Read the model definition and answer for the solid it produces. Units are mm, in the model's axes. A direction names the side the tool comes from. Coordinates: 2 decimals unless noted, no trailing zeros. Write each loop counter-clockwise with the first axis right and the second up, starting at its lowest first coordinate (ties: lowest second). Pieces come first, ordered by that corner, then holes. Notation, with made-up numbers: (59, 62) -> (83, 62) arc R6 cw to (83, 71) -> close; hole circle Ø11 at (20.5, 62). An arc over 180 degrees is marked (long way). One line per item, written item: value. Start each with the question number.
1. Consider line 1 along Y through (x, z) = (11, 3.5); line 2 along Y through (x, z) = (3.75, 0.5); line 3 along Z through (x, y) = (-0.75, 14.75). Determine where each line is inside the solid, lowest interval first.
2. Given P1, Ø4, axis at x = -4.5, z = 2, coming from the +Y side; P2, Ø2.5, axis at y = 18, z = 3.5, coming from the +X side; P3, Ø3, axis at x = 7.5, z = 4, coming from the +Y side, each flat-ended and moving along its own axis, determine where each tip first touches the part or whether it passes through.
3. Find section D-D, the plane z = -2. Write down the section's boundary in (x, y).
4. Find section A-A, the plane z = 4. Write down the section's boundary in (x, y).
5. Find section B-B, the plane x = 3. Write down the section's boundary in (y, z), and give its area (3 significant figures).
6. For faces 1 (the flat face through (4.965, 7.465, 2.605)), 2 (the flat face through (-12.5, 10, 0)), determine the directions among +Z, -Z, +X, -X, +Y, -Y from which every point of the face is accessible in a straight line to the end or side of a thin tool.
7. Find section C-C, the plane y = 6. Write down the section's boundary in (x, z), and give its area (4 significant figures).
```python
from build123d import *

# Parameters (mm, degrees)
SKETCH_1_W          = 5
SKETCH_1_H          = 15
EXTRUDE_1_DEPTH     = 5
EXTRUDE_2_DEPTH     = 10
SKETCH_1_4_W        = 5
SKETCH_1_4_H        = 15
EXTRUDE_3_DEPTH     = 15
EXTRUDE_4_DEPTH     = 20
CUT_EXTRUDE_1_DEPTH = 20


with BuildPart() as part:
    # Sketch 1 → Extrude 1 (new body)
    with BuildSketch(Plane(origin=(0, 0, 0), x_dir=(1, 0, 0), z_dir=(0, 1, 0))):
        Polygon((7.5, 5), (12.5, 5), (12.5, 10), (-12.5, 10), (-12.5, -10), (-7.5, -10), (-7.5, 5), (-2.5, 5), align=None)
        with Locations((-5, -2.5)):
            Rectangle(SKETCH_1_W, SKETCH_1_H)
        Polygon((2.5, -10), (7.5, 5), (-2.5, 5), (-2.5, -10), align=None)
        Polygon((12.5, -10), (12.5, 5), (7.5, 5), (2.5, -10), align=None)
    extrude(amount=EXTRUDE_1_DEPTH)

    # Sketch 1_3 → Extrude 2 (add)
    with BuildSketch(Plane(origin=(0, 0, 0), x_dir=(1, 0, 0), z_dir=(0, 1, 0))):
        Polygon((2.5, -10), (7.5, 5), (-2.5, 5), (-2.5, -10), align=None)
    extrude(amount=EXTRUDE_2_DEPTH)

    # Sketch 1_4 → Extrude 3 (add)
    with BuildSketch(Plane(origin=(0, 0, 0), x_dir=(1, 0, 0), z_dir=(0, 1, 0))):
        with Locations((-5, -2.5)):
            Rectangle(SKETCH_1_4_W, SKETCH_1_4_H)
    extrude(amount=EXTRUDE_3_DEPTH)

    # Sketch 1_5 → Extrude 4 (add)
    with BuildSketch(Plane(origin=(0, 0, 0), x_dir=(1, 0, 0), z_dir=(0, 1, 0))):
        Polygon((7.5, 5), (12.5, 5), (12.5, 10), (-12.5, 10), (-12.5, -10), (-7.5, -10), (-7.5, 5), (-2.5, 5), align=None)
    extrude(amount=EXTRUDE_4_DEPTH)

    # Sketch 2 → Cut-Extrude 1 (cut)
    with BuildSketch(Plane.XY.offset(-5)):
        Polygon((12.5, 20), (2.5, 20), (12.5, 10), align=None)
    extrude(amount=-CUT_EXTRUDE_1_DEPTH, mode=Mode.SUBTRACT)


solid = part.part
```
Answer block:
1. line 1: y = 0 to 5
1. line 2: y = 0 to 10
1. line 3: z = -10 to -5
2. P1: stops at y = 15
2. P2: stops at x = -7.5
2. P3: stops at y = 5
3. outline: (-12.5, 0) -> (12.5, 0) -> (12.5, 5) -> (6.5, 5) -> (6.5, 10) -> (-2.5, 10) -> (-2.5, 15) -> (-7.5, 15) -> (-7.5, 20) -> (-12.5, 20) -> close
4. outline: (-12.5, 0) -> (12.5, 0) -> (12.5, 5) -> (4.5, 5) -> (4.5, 10) -> (-2.5, 10) -> (-2.5, 15) -> (-7.5, 15) -> (-7.5, 20) -> (-12.5, 20) -> close
5. outline: (0, -10) -> (19.5, -10) -> (19.5, -5) -> (10, -5) -> (10, 8.5) -> (5, 8.5) -> (5, 10) -> (0, 10) -> close
5. area: 240 mm2
6. face 1: +Z, +X, +Y
6. face 2: +Z, -Z, -X, +Y, -Y
7. outline: (-12.5, -10) -> (12.5, -10) -> (12.5, -5) -> (7.5, -5) -> (2.5, 10) -> (-12.5, 10) -> close
7. area: 387.5 mm2
